Verification items for the finished model (mm, model axes). A direction names the side the tool comes from. Coordinates: 2 decimals unless noted, no trailing zeros. Loops run counter-clockwise (first coordinate to the right, second up) from the corner with the lowest first, then second, coordinate; pieces in that order, holes last. Notation, with made-up numbers: (89.25, -17.5) -> (129.25, -17.5) arc R25 ccw to (129.25, 21.5) -> close; hole circle Ø3 at (52.5, -26.75). An arc over 180 degrees is marked (long way). Write item = value, one per line.
```python
from build123d import *


with BuildPart() as part:
    # Szkic1 → Obrót1 (revolve)
    with BuildSketch(Plane.XY, mode=Mode.PRIVATE) as obr_t1_sk:
        with BuildLine():
            Line((0, 0), (6, 0))
            Line((6, 0), (6, -1))
            Line((6, -1), (5, -2))
            Line((5, -2), (4, -2))
            ThreePointArc((4, -2), (3.292893219, -2.292893219), (3, -3))
            Line((3, -3), (3, -6))
            Line((3, -6), (1.5, -6))
            ThreePointArc((1.5, -6), (1.060660172, -4.939339828), (0, -4.5))
            Line((0, -4.5), (0, 0))
        make_face()
    revolve(obr_t1_sk.sketch.rotate(Axis((0, -4.5, 0), (0, 1, 0)), 90), axis=Axis((0, -4.5, 0), (0, 1, 0)))


solid = part.part
```
1) Sectioned sample at A-A, the plane x = 0. Record the cut outline in (y, z).
Ans:
outline = (-6, -3) -> (-3, -3) arc R1 cw to (-2, -4) -> (-2, -5) -> (-1, -6) -> (0, -6) -> (0, 6) -> (-1, 6) -> (-2, 5) -> (-2, 4) arc R1 cw to (-3, 3) -> (-6, 3) -> (-6, 1.5) arc R1.5 cw to (-6, -1.5) -> close
2) Sectioned sample at B-B, the plane z = 0. Record the cut outline in (x, y), plus the area to 3 significant figures.
Ans:
outline = (-6, -1) -> (-5, -2) -> (-4, -2) arc R1 cw to (-3, -3) -> (-3, -6) -> (-1.5, -6) arc R1.5 cw to (1.5, -6) -> (3, -6) -> (3, -3) arc R1 cw to (4, -2) -> (5, -2) -> (6, -1) -> (6, 0) -> (-6, 0) -> close
area = 43.9 mm2
3) Material ranges on line 1 (Y direction, x = -3, z = 2.5); line 2 (Z direction, x = 3.5, y = -0.8); line 3 (Y direction, x = 1.25, z = 5), recorded low to high.
Ans:
line_1 = -2 to 0
line_2 = -4.87 to 4.87
line_3 = -1.85 to 0
4) Sectioned sample at D-D, the plane y = -5. Record the cut outline in (x, z).
Ans:
outline = circle Ø6 at (0, 0); hole circle Ø2.24 at (0, 0)
5) Sectioned sample at C-C, the plane y = -1.2. Record the cut outline in (x, z), plus the area to 3 significant figures.
Ans:
outline = circle Ø11.6 at (0, 0)
area = 106 mm2
6) Tool access check on faces 1 (the face through (-0.9, -4.52, -2.86)), 2 (the face through (0, 0, 0)). Record the directions out of +Z, -Z, +X, -X, +Y, -Y that give a thin tool (end or side, any length) a straight path to the whole face; none if there is none.
Ans:
face_1 = -Y
face_2 = +Z, -Z, +X, -X, +Y
7) Depth check by flat-ended pin: pin 1 Ø1 at (x, y) = (-0.5, -2) entering from +Z; pin 2 Ø1.5 at (x, y) = (0, -4) entering from +Z; pin 3 Ø3 at (x, y) = (4.5, -1) entering from -Z. Enter the tip coordinate at first touch or a pass-through.
Ans:
pin_1 = 5.48
pin_2 = 3
pin_3 = -5.2
